Read the model definition and answer for the solid it produces. Units are mm, in the model's axes. A direction names the side the tool comes from. Give positions to 0.01 mm unless a question says otherwise; leave off trailing zeros. Loops run counter-clockwise (first coordinate to the right, second up) from the corner with the lowest first, then second, coordinate; pieces in that order, holes last.
(1) Find section D-D, the plane x = -14.5. Write down the section's boundary in (y, z), then the cut area to 3 significant figures.
(2) Straight lines are drawn through the part: probe 1 along Z at (x, y) = (-10, -35); probe 2 along Y at (x, z) = (-18, 210); probe 3 along X at (y, z) = (29.5, 261). For each, find the intervals that lie inside material, in ascending order.
(3) Find section A-A, the plane x = 0. Write down the section's boundary in (y, z), then the cut area to 3 significant figures.
(4) Find section B-B, the plane y = 0. Write down the section's boundary in (x, z).
(5) Which of the six approach directions +Z, -Z, +X, -X, +Y, -Y give full straight-line access (tool end or side, diameter ignored) to faces 1 (the face through (35, 0, 0)), 2 (the face through (37, 0, 12)), 3 (the face through (-32, -48, 260))?
(6) Determine the mould class of faces 4 (the face through (-37, 0, 12)), 5 (the face through (-12.26, -0.67, 279.56)), 6 (the face through (1.32, -1.15, -29.97)) for opening direction X: pulls with the +X half, pulls with the -X half, needs draft (parallel to the pull), parting line crosses it, or undercut.
(7) Find section C-C, the plane z = 205. Write down the section's boundary in (x, y).
(8) Each of these flat-tipped pins is pushed along its axis until it touches: P1, Ø12.5, axis at x = -35, y = -12, coming from the +Z side; P2, Ø6.5, axis at x = -38, y = -15, coming from the -Z side; P3, Ø1.5, axis at y = -8.5, z = 23, coming from the +X side. Where does it stop, or does it pass through?
```python
from build123d import *

# Parameters (mm, degrees)
EXTRUDE_1_DEPTH      = 82
EXTRUDE_1_DEPTH_BACK = 82
SKETCH_1_R           = 30
SKETCH_2_R           = 43
EXTRUDE_2_DEPTH      = 12
SKETCH_3_R           = 36
EXTRUDE_3_DEPTH      = 250
EXTRUDE_5_DEPTH      = 48
EXTRUDE_5_DEPTH_BACK = 48
SKETCH_5_R           = 49
SKETCH_5_R_2         = 32


with BuildPart() as part:
    # Sketch 1 → Extrude 1 (new, two sides: drawn at the far end of the back side and taken through both)
    with BuildSketch(Plane(origin=(0, 0, 0), x_dir=(1, 0, 0), z_dir=(0, 1, 0)).offset(-EXTRUDE_1_DEPTH_BACK)):
        with Locations(Location((0, 0, 0), (0, 0, 270))):
            Circle(SKETCH_1_R)
    extrude(amount=EXTRUDE_1_DEPTH + EXTRUDE_1_DEPTH_BACK)

    # Sketch 2 → Extrude 2 (add)
    with BuildSketch(Plane.XY):
        Circle(SKETCH_2_R)
    extrude(amount=EXTRUDE_2_DEPTH)

    # Sketch 3 → Extrude 3 (add)
    with BuildSketch(Plane.XY):
        with Locations(Location((0, 0, 0), (0, 0, 139.797034655))):
            Circle(SKETCH_3_R)
    extrude(amount=EXTRUDE_3_DEPTH)

    # Sketch 5 → Extrude 5 (add, two sides: drawn at the far end of the back side and taken through both)
    with BuildSketch(Plane(origin=(0, 0, 0), x_dir=(1, 0, 0), z_dir=(0, 1, 0)).offset(-EXTRUDE_5_DEPTH_BACK)):
        with Locations(Location((0, -250, 0), (0, 0, 270))):
            Circle(SKETCH_5_R)
        with Locations(Location((0, -250, 0), (0, 0, 270))):
            Circle(SKETCH_5_R_2, mode=Mode.SUBTRACT)
    extrude(amount=EXTRUDE_5_DEPTH + EXTRUDE_5_DEPTH_BACK)


solid = part.part
```
Entries:
1. outline: (-82, -26.26) - (82, -26.26) - (82, 26.26) - (32.95, 26.26) - (32.95, 203.19) - (48, 203.19) - (48, 221.47) - (32.95, 221.47) - (32.95, 250) - (-32.95, 250) - (-32.95, 221.47) - (-48, 221.47) - (-48, 203.19) - (-32.95, 203.19) - (-32.95, 26.26) - (-82, 26.26) - close; (-48, 278.53) - (48, 278.53) - (48, 296.81) - (-48, 296.81) - close
1. area: 25,700 mm2
2. probe 1: z = -28.28 to 28.28, 202.03 to 219.6, 280.4 to 297.97
2. probe 2: y = -48 to 48
2. probe 3: x = -47.75 to -30.05, 30.05 to 47.75
3. outline: (-82, -30) - (82, -30) - (82, 30) - (36, 30) - (36, 201) - (48, 201) - (48, 218) - (36, 218) - (36, 250) - (-36, 250) - (-36, 218) - (-48, 218) - (-48, 201) - (-36, 201) - (-36, 30) - (-82, 30) - close; (-48, 282) - (48, 282) - (48, 299) - (-48, 299) - close
3. area: 27,700 mm2
4. outline: (-43, 0) - (-30, 0) arc R30 ccw to (30, 0) - (43, 0) - (43, 12) - (36, 12) - (36, 216.76) arc R49 ccw (long way) to (-36, 216.76) - (-36, 12) - (-43, 12) - close; hole (-32, 250) - (32, 250) arc R32 ccw to start
5. face 1: -Z, +X, +Y, -Y
5. face 2: +X
5. face 3: +Z, +X, -X, -Y
6. face 4: needs draft
6. face 5: undercut
6. face 6: parting line crosses it
7. outline: (-19.39, -48) - (19.39, -48) - (19.39, -30.33) arc R36 ccw to (19.39, 30.33) - (19.39, 48) - (-19.39, 48) - (-19.39, 30.33) arc R36 ccw to (-19.39, -30.33) - close
8. P1: stops at z = 289.68
8. P2: stops at z = 0
8. P3: stops at x = 35.16
